from build123d import *

# Parameters (mm, degrees)
SKETCH1_R           = 25
SKETCH1_R_2         = 4
BOSS_EXTRUDE1_DEPTH = 2.5
SKETCH4_R           = 10.5
CUT_EXTRUDE3_DEPTH  = 2
CUT_EXTRUDE2_REACH  = 37.707
SKETCH3_R           = 1.65
FILLET1_R           = 0.5
CUT_EXTRUDE4_REACH  = 37.482
SKETCH5_R           = 1.65


with BuildPart() as part:
    # Sketch1 → Boss-Extrude1 (new, symmetric)
    with BuildSketch(Plane(origin=(0, 0, 0), x_dir=(1, 0, 0), z_dir=(0, 1, 0))):
        with Locations(Location((0, 0, 0), (0, 0, 270))):
            Circle(SKETCH1_R)
        with Locations(Location((0, 0, 0), (0, 0, 270))):
            Circle(SKETCH1_R_2, mode=Mode.SUBTRACT)
    extrude(amount=BOSS_EXTRUDE1_DEPTH, both=True)

    # Sketch4 → Cut-Extrude3 (cut)
    with BuildSketch(Plane(origin=(0, 2.5, 0), x_dir=(1, 0, 0), z_dir=(0, 1, 0))):
        with Locations(Location((0, 0, 0), (0, 0, 270))):
            Circle(SKETCH4_R)
    extrude(amount=-CUT_EXTRUDE3_DEPTH, mode=Mode.SUBTRACT)

    # Sketch3 → Cut-Extrude2 (cut, up to next)
    with BuildSketch(Plane.XZ.offset(2.5), mode=Mode.PRIVATE) as cut_extrude2_sk1:
        with Locations(Location((-15, 15, 0), (0, 0, 270))):
            Circle(SKETCH3_R)
    cut_extrude2_tool1 = extrude(cut_extrude2_sk1.sketch, amount=-CUT_EXTRUDE2_REACH, mode=Mode.PRIVATE) & part.part
    # Sketch3 → Cut-Extrude2 (cut, up to next)
    with BuildSketch(Plane.XZ.offset(2.5), mode=Mode.PRIVATE) as cut_extrude2_sk2:
        with Locations(Location((15, 15, 0), (0, 0, 270))):
            Circle(SKETCH3_R)
    cut_extrude2_tool2 = extrude(cut_extrude2_sk2.sketch, amount=-CUT_EXTRUDE2_REACH, mode=Mode.PRIVATE) & part.part
    # Sketch3 → Cut-Extrude2 (cut, up to next)
    with BuildSketch(Plane.XZ.offset(2.5), mode=Mode.PRIVATE) as cut_extrude2_sk3:
        with Locations(Location((15, -15, 0), (0, 0, 270))):
            Circle(SKETCH3_R)
    cut_extrude2_tool3 = extrude(cut_extrude2_sk3.sketch, amount=-CUT_EXTRUDE2_REACH, mode=Mode.PRIVATE) & part.part
    # Sketch3 → Cut-Extrude2 (cut, up to next)
    with BuildSketch(Plane.XZ.offset(2.5), mode=Mode.PRIVATE) as cut_extrude2_sk4:
        with Locations(Location((-15, -15, 0), (0, 0, 270))):
            Circle(SKETCH3_R)
    cut_extrude2_tool4 = extrude(cut_extrude2_sk4.sketch, amount=-CUT_EXTRUDE2_REACH, mode=Mode.PRIVATE) & part.part
    # Sketch3 → Cut-Extrude2 (cut, up to next)
    with BuildSketch(Plane.XZ.offset(2.5), mode=Mode.PRIVATE) as cut_extrude2_sk5:
        with Locations(Location((0, 15, 0), (0, 0, 270))):
            Circle(SKETCH3_R)
    cut_extrude2_tool5 = extrude(cut_extrude2_sk5.sketch, amount=-CUT_EXTRUDE2_REACH, mode=Mode.PRIVATE) & part.part
    # Sketch3 → Cut-Extrude2 (cut, up to next)
    with BuildSketch(Plane.XZ.offset(2.5), mode=Mode.PRIVATE) as cut_extrude2_sk6:
        with Locations(Location((15, 0, 0), (0, 0, 270))):
            Circle(SKETCH3_R)
    cut_extrude2_tool6 = extrude(cut_extrude2_sk6.sketch, amount=-CUT_EXTRUDE2_REACH, mode=Mode.PRIVATE) & part.part
    # Sketch3 → Cut-Extrude2 (cut, up to next)
    with BuildSketch(Plane.XZ.offset(2.5), mode=Mode.PRIVATE) as cut_extrude2_sk7:
        with Locations(Location((0, -15, 0), (0, 0, 270))):
            Circle(SKETCH3_R)
    cut_extrude2_tool7 = extrude(cut_extrude2_sk7.sketch, amount=-CUT_EXTRUDE2_REACH, mode=Mode.PRIVATE) & part.part
    # Sketch3 → Cut-Extrude2 (cut, up to next)
    with BuildSketch(Plane.XZ.offset(2.5), mode=Mode.PRIVATE) as cut_extrude2_sk8:
        with Locations(Location((-15, 0, 0), (0, 0, 270))):
            Circle(SKETCH3_R)
    cut_extrude2_tool8 = extrude(cut_extrude2_sk8.sketch, amount=-CUT_EXTRUDE2_REACH, mode=Mode.PRIVATE) & part.part
    add(cut_extrude2_tool1.solids().sort_by_distance((-15, -2.5, 15))[0], mode=Mode.SUBTRACT)
    add(cut_extrude2_tool2.solids().sort_by_distance((15, -2.5, 15))[0], mode=Mode.SUBTRACT)
    add(cut_extrude2_tool3.solids().sort_by_distance((15, -2.5, -15))[0], mode=Mode.SUBTRACT)
    add(cut_extrude2_tool4.solids().sort_by_distance((-15, -2.5, -15))[0], mode=Mode.SUBTRACT)
    add(cut_extrude2_tool5.solids().sort_by_distance((0, -2.5, 15))[0], mode=Mode.SUBTRACT)
    add(cut_extrude2_tool6.solids().sort_by_distance((15, -2.5, 0))[0], mode=Mode.SUBTRACT)
    add(cut_extrude2_tool7.solids().sort_by_distance((0, -2.5, -15))[0], mode=Mode.SUBTRACT)
    add(cut_extrude2_tool8.solids().sort_by_distance((-15, -2.5, 0))[0], mode=Mode.SUBTRACT)

    # Fillet1
    fillet1_edges = [part.edges().sort_by_distance(p)[0] for p in [
        (0, 2.5, -10.5),
        (0, -2.5, -25),
        (0, 2.5, -25),
    ]]
    fillet(fillet1_edges, radius=FILLET1_R)

    # Sketch5 → Cut-Extrude4 (cut, up to next)
    with BuildSketch(Plane(origin=(0, 0.5, 0), x_dir=(1, 0, 0), z_dir=(0, 1, 0)), mode=Mode.PRIVATE) as cut_extrude4_sk1:
        with Locations(Location((0, 7, 0), (0, 0, 270))):
            Circle(SKETCH5_R)
    cut_extrude4_tool1 = extrude(cut_extrude4_sk1.sketch, amount=-CUT_EXTRUDE4_REACH, mode=Mode.PRIVATE) & part.part
    # Sketch5 → Cut-Extrude4 (cut, up to next)
    with BuildSketch(Plane(origin=(0, 0.5, 0), x_dir=(1, 0, 0), z_dir=(0, 1, 0)), mode=Mode.PRIVATE) as cut_extrude4_sk2:
        with Locations(Location((0, -7, 0), (0, 0, 270))):
            Circle(SKETCH5_R)
    cut_extrude4_tool2 = extrude(cut_extrude4_sk2.sketch, amount=-CUT_EXTRUDE4_REACH, mode=Mode.PRIVATE) & part.part
    # Sketch5 → Cut-Extrude4 (cut, up to next)
    with BuildSketch(Plane(origin=(0, 0.5, 0), x_dir=(1, 0, 0), z_dir=(0, 1, 0)), mode=Mode.PRIVATE) as cut_extrude4_sk3:
        with Locations(Location((7, 0, 0), (0, 0, 270))):
            Circle(SKETCH5_R)
    cut_extrude4_tool3 = extrude(cut_extrude4_sk3.sketch, amount=-CUT_EXTRUDE4_REACH, mode=Mode.PRIVATE) & part.part
    # Sketch5 → Cut-Extrude4 (cut, up to next)
    with BuildSketch(Plane(origin=(0, 0.5, 0), x_dir=(1, 0, 0), z_dir=(0, 1, 0)), mode=Mode.PRIVATE) as cut_extrude4_sk4:
        with Locations(Location((-7, 0, 0), (0, 0, 270))):
            Circle(SKETCH5_R)
    cut_extrude4_tool4 = extrude(cut_extrude4_sk4.sketch, amount=-CUT_EXTRUDE4_REACH, mode=Mode.PRIVATE) & part.part
    add(cut_extrude4_tool1.solids().sort_by_distance((0, 0.5, -7))[0], mode=Mode.SUBTRACT)
    add(cut_extrude4_tool2.solids().sort_by_distance((0, 0.5, 7))[0], mode=Mode.SUBTRACT)
    add(cut_extrude4_tool3.solids().sort_by_distance((7, 0.5, 0))[0], mode=Mode.SUBTRACT)
    add(cut_extrude4_tool4.solids().sort_by_distance((-7, 0.5, 0))[0], mode=Mode.SUBTRACT)


solid = part.part
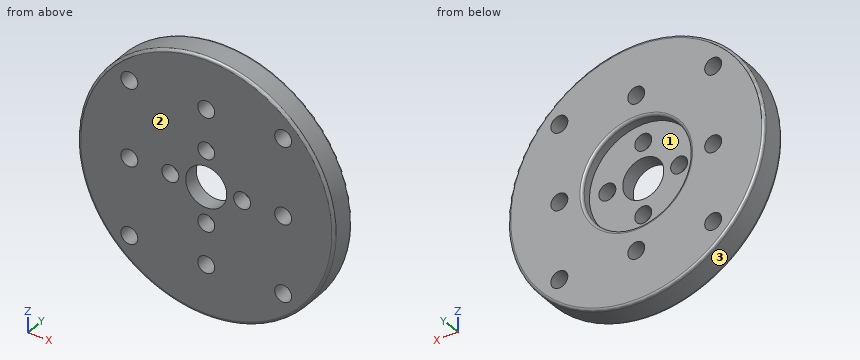
Input: part model. Units: mm. Frame: model coordinates. Face numbers are marked on the shaded views. Round coordinates to 2 decimals unless told otherwise and drop trailing zeros. Answer as a JSON object with one key per item and string values. Group by question number.
1) Pin query (flat end, axial travel): pin 1 (1.5 mm diameter, centred on y = -2, z = 1.5, fed in from -X); pin 2 (4.5 mm diameter, centred on x = 15, z = -15, fed in from -Y); pin 3 (1.5 mm diameter, centred on y = 0, z = 14, fed in from -X); pin 4 (2.5 mm diameter, centred on x = 15, z = 15, fed in from -Y). Return the tip coordinate at first contact, or that it passes through.
2) Section query A-A on y = -1.4. State how many separate pieces and enclosed holes the cut face has, plus the area to 3 significant figures.
3) Draft query along Z for the marked faces 1, 2 and 3. Return one class per face: +Z half, -Z half, draft (parallel to the pull), parting line (faces both ways), or undercut.
4) Ray query, L1, parallel to X at y = -1.3, z = 0; L2, parallel to X at y = 1.25, z = 0; L3, parallel to X at y = -0.4, z = -1. Return the intervals inside material, ascending.
Reply:
{
 "1": {"pin 1": "stops at x = -24.99", "pin 2": "stops at y = -2.5", "pin 3": "stops at x = -21.2", "pin 4": "passes through"},
 "2": {"separate pieces": "1", "enclosed holes": "13", "area": "1,810 mm2"},
 "3": {"face 1": "undercut", "face 2": "draft", "face 3": "parting line"},
 "4": {"L1": "x = -25 to -16.65, -13.35 to -8.65, -5.35 to -4, 4 to 5.35, 8.65 to 13.35, 16.65 to 25", "L2": "x = -25 to -16.65, -13.35 to -10.5, 10.5 to 13.35, 16.65 to 25", "L3": "x = -24.98 to -16.31, -13.69 to -8.31, -5.69 to -3.87, 3.87 to 5.69, 8.31 to 13.69, 16.31 to 24.98"}
}
